Read the model definition and answer for the solid it produces. Units are mm, in the model's axes. A direction names the side the tool comes from. Coordinates: 2 decimals unless noted, no trailing zeros. Write each loop counter-clockwise with the first axis right and the second up, starting at its lowest first coordinate (ties: lowest second). Pieces come first, ordered by that corner, then holes.
(1) The part is cut by section B-B, the plane y = 24. State how many separate pieces and enclosed holes the cut face has, and give its area (3 significant figures).
(2) The part is cut by section A-A, the plane z = 0. Determine the outline of the cut face in (x, y) (3 decimals), and give its area (3 significant figures).
(3) Determine the mould class of faces 3 (the flat face through (0, 32, 0)), 4 (the flat face through (44.347, 1.513, 17.306)), 5 (the cylindrical face through (69.09, 1.08, 0.99)) for opening direction X: pulls with the +X half, pulls with the -X half, needs draft (parallel to the pull), parting line crosses it, or undercut.
(4) Given pin 1 (6 mm diameter, centred on y = 56.5, z = -9.5, fed in from +X); pin 2 (3.5 mm diameter, centred on y = 24, z = 13.5, fed in from +X) (3 decimals); pin 3 (4 mm diameter, centred on x = 23, z = -5.5, fed in from +Y), each flat-ended and moving along its own axis, determine where each tip first touches the part or whether it passes through.
(5) Which of the six approach directions +Z, -Z, +X, -X, +Y, -Y give full straight-line access (tool end or side, diameter ignored) to faces 1 (the cylindrical face through (3.71, 44.27, 17.01)), 2 (the flat face through (4, 34, 0))?
(6) Straight lines are drawn through the part: line 1 along X through (y, z) = (39.5, 9); line 2 along X through (y, z) = (1.3, 0). For each, find the intervals that lie inside material, in ascending order.
```python
from build123d import *

# Parameters (mm, degrees)
EXTRUDE_THIN2_DEPTH = 25.9953125
CUT_EXTRUDE1_DEPTH  = 114.59781347
CUT_EXTRUDE2_DEPTH  = 114.59781347
SKETCH5_R           = 2.15
CUT_EXTRUDE4_DEPTH  = 114.59781347
SKETCH4_R           = 2.15
CUT_EXTRUDE3_DEPTH  = 114.59781347
FILLET1_R           = 1.016
FILLET2_R           = 1.905
CHAMFER1_SIZE       = 1.8796


with BuildPart() as part:
    # Sketch1 → Extrude-Thin2 (new, symmetric)
    with BuildSketch(Plane.XY):
        with BuildLine():
            Line((80.16875, 0), (1.905, 0))
            ThreePointArc((1.905, 0), (0.557961582, 0.557961582), (0, 1.905))
            Line((0, 1.905), (0, 80.16875))
            Line((0, 80.16875), (4, 80.16875))
            Line((4, 80.16875), (4, 4))
            Line((4, 4), (80.16875, 4))
            Line((80.16875, 4), (80.16875, 0))
        make_face()
    extrude(amount=EXTRUDE_THIN2_DEPTH, both=True)

    # Sketch2 → Cut-Extrude1 (cut, through all)
    with BuildSketch(Plane(origin=(4, 0, 0), x_dir=(0, 0, -1), z_dir=(1, 0, 0))):
        Polygon((-8.5, 80.16875), (8.5, 80.16875), (25.9953125, 9), (38.1, 9), (38.1, 105.56875), (-38.1, 105.56875), (-38.1, 9), (-25.9953125, 9), align=None)
    extrude(amount=-CUT_EXTRUDE1_DEPTH, mode=Mode.SUBTRACT)

    # Sketch3 → Cut-Extrude2 (cut, through all)
    with BuildSketch(Plane(origin=(0, 4, 0), x_dir=(1, 0, 0), z_dir=(0, 1, 0))):
        Polygon((9, 25.9953125), (80.16875, 8.5), (80.16875, -8.5), (9, -25.9953125), (9, -38.1), (105.56875, -38.1), (105.56875, 38.1), (9, 38.1), align=None)
    extrude(amount=-CUT_EXTRUDE2_DEPTH, mode=Mode.SUBTRACT)

    # Sketch5 → Cut-Extrude4 (cut, through all)
    with BuildSketch(Plane(origin=(0, 4, 0), x_dir=(1, 0, 0), z_dir=(0, 1, 0))):
        with Locations(Location((71, 0, 0), (0, 0, 270))):
            Circle(SKETCH5_R)
        with Locations(Location((24, 13.5, 0), (0, 0, 270))):
            Circle(SKETCH5_R)
        with Locations(Location((24, -13.5, 0), (0, 0, 90))):
            Circle(SKETCH5_R)
    extrude(amount=-CUT_EXTRUDE4_DEPTH, mode=Mode.SUBTRACT)

    # Sketch4 → Cut-Extrude3 (cut, through all)
    with BuildSketch(Plane(origin=(4, 0, 0), x_dir=(0, 0, -1), z_dir=(1, 0, 0))):
        with Locations((0, 71)):
            Circle(SKETCH4_R)
        with Locations((-13.5, 24)):
            Circle(SKETCH4_R)
        with Locations(Location((13.5, 24, 0), (0, 0, 180))):
            Circle(SKETCH4_R)
    extrude(amount=-CUT_EXTRUDE3_DEPTH, mode=Mode.SUBTRACT)

    # Fillet1
    fillet1_edges = [part.edges().sort_by_distance(p)[0] for p in [
        (6.5, 4, 25.9953125),
        (4, 4, 0),
        (4, 6.5, -25.9953125),
        (4, 6.5, 25.9953125),
        (4, 80.16875, 0),
        (4, 44.584375, 17.24765625),
        (4, 44.584375, -17.24765625),
        (80.16875, 4, 0),
        (44.584375, 4, 17.24765625),
        (44.584375, 4, -17.24765625),
        (6.5, 4, -25.9953125),
    ]]
    fillet(fillet1_edges, radius=FILLET1_R)

    # Fillet2
    # the kernel refuses this fillet: 1.905 mm, written as the material it takes off along each edge
    with BuildSketch(Plane(origin=(78.26375, 4, 7.00658656), x_dir=(0.23872121575662697, 0, 0.9710881428313695), z_dir=(-0.9710881428313695, 0, 0.23872121575662697))) as fillet2_piece_1:
        with BuildLine():
            CenterArc((0.889, -1.016), 1.016, 0, 90)
            Line((1.905, -1.016), (1.905, 0))
            Line((1.905, 0), (0.889, 0))
        make_face()
    revolve(axis=Axis((78.26375, 4, 7.00658656), (0, 1, 0)), revolution_arc=76.188922225, mode=Mode.SUBTRACT)
    with BuildSketch(Plane(origin=(4, 78.26375, 7.00658656), x_dir=(0, 1, 0), z_dir=(0, 0, -1))) as fillet2_piece_2:
        with BuildLine():
            CenterArc((0.889, -1.016), 1.016, 0, 90)
            Line((1.905, -1.016), (1.905, 0))
            Line((1.905, 0), (0.889, 0))
        make_face()
    revolve(axis=Axis((4, 78.26375, 7.00658656), (1, 0, 0)), revolution_arc=76.188922225, mode=Mode.SUBTRACT)
    with BuildSketch(Plane(origin=(4, 78.26375, -7.00658656), x_dir=(0, 0.23872121575662691, -0.9710881428313693), z_dir=(0, -0.9710881428313693, -0.23872121575662691))) as fillet2_piece_3:
        with BuildLine():
            CenterArc((0.889, -1.016), 1.016, 0, 90)
            Line((1.905, -1.016), (1.905, 0))
            Line((1.905, 0), (0.889, 0))
        make_face()
    revolve(axis=Axis((4, 78.26375, -7.00658656), (1, 0, 0)), revolution_arc=76.188922225, mode=Mode.SUBTRACT)
    with BuildSketch(Plane(origin=(78.26375, 4, -7.00658656), x_dir=(1, 0, 0), z_dir=(0, 0, 1))) as fillet2_piece_4:
        with BuildLine():
            CenterArc((0.889, -1.016), 1.016, 0, 90)
            Line((1.905, -1.016), (1.905, 0))
            Line((1.905, 0), (0.889, 0))
        make_face()
    revolve(axis=Axis((78.26375, 4, -7.00658656), (0, 1, 0)), revolution_arc=76.188922225, mode=Mode.SUBTRACT)
    with BuildSketch(Plane(origin=(4, 80.16875, 8.5), x_dir=(0, -0.971088142831369, 0.23872121575662839), z_dir=(-1, 0, 0)), Plane(origin=(80.16875, 4, 8.5), x_dir=(0, 0, -1), z_dir=(0, -1, 0))) as fillet2_piece_5:
        with BuildLine():
            CenterArc((FILLET2_R * 0.783944063022, -FILLET2_R), FILLET2_R, 90, 76.188922225)
            Line((-FILLET2_R * 0.18714407981, -FILLET2_R * 0.761278784243), (0, 0))
            Line((0, 0), (FILLET2_R * 0.783944063022, 0))
        make_face()
    extrude(amount=7.7335336, mode=Mode.SUBTRACT)
    with BuildSketch(Plane(origin=(4, 80.16875, -8.5), x_dir=(0, -0.9710881428313692, -0.23872121575662728), z_dir=(-1, 0, 0)), Plane(origin=(80.16875, 4, -8.5), x_dir=(0, 0, 1), z_dir=(0, -1, 0))) as fillet2_piece_6:
        with BuildLine():
            CenterArc((FILLET2_R * 0.783944063022, FILLET2_R), FILLET2_R, 193.811077775, 76.188922225)
            Line((-FILLET2_R * 0.18714407981, FILLET2_R * 0.761278784243), (0, 0))
            Line((0, 0), (FILLET2_R * 0.783944063022, 0))
        make_face()
    extrude(amount=7.7335336, mode=Mode.SUBTRACT)

    # Chamfer1
    chamfer1_edges = [part.edges().sort_by_distance(p)[0] for p in [
        (71, 4, -2.15),
        (24, 4, -15.65),
        (24, 4, 15.65),
        (4, 71, 2.15),
        (4, 24, 15.65),
        (4, 24, -15.65),
    ]]
    chamfer(chamfer1_edges, length=CHAMFER1_SIZE)


solid = part.part
```
Computed:
1. separate pieces: 3
1. enclosed holes: 0
1. area: 137 mm2
2. outline: (0, 1.905) arc R1.905 ccw to (1.905, 0) - (68.85, 0) - (68.85, 2.12) - (66.97, 4) - (5.016, 4) arc R1.016 cw to (4, 5.016) - (4, 66.97) - (2.12, 68.85) - (0, 68.85) - close; (0, 73.15) - (2.12, 73.15) - (4, 75.03) - (4, 79.153) arc R1.016 ccw to (2.984, 80.169) - (0, 80.169) - close; (73.15, 0) - (80.169, 0) - (80.169, 2.984) arc R1.016 ccw to (79.153, 4) - (75.03, 4) - (73.15, 2.12) - close
2. area: 583 mm2
3. face 3: pulls with the -X half
3. face 4: pulls with the +X half
3. face 5: undercut
4. pin 1: stops at x = 4
4. pin 2: passes through
4. pin 3: stops at y = 4
5. face 1: +Z, +X, +Y
5. face 2: +Z, -Z, +X, +Y
6. line 1: x = 0 to 4
6. line 2: x = 0.1 to 68.85, 73.15 to 80.17
